Read the model definition and answer for the solid it produces. Units are mm, in the model's axes. A direction names the side the tool comes from. Coordinates: 2 decimals unless noted, no trailing zeros. Write each loop counter-clockwise with the first axis right and the second up, starting at its lowest first coordinate (ties: lowest second). Pieces come first, ordered by that corner, then holes.
Item 1: A tool of negligible diameter and unlimited length cuts with its end or side. For faces 1 (the face through (30, 6, -66.1)), 2 (the face through (73.379, 5.944, -44.985)), 3 (the face through (49, 10, -2)), from which of +Z, -Z, +X, -X, +Y, -Y can it reach the whole face along a straight path? Write none if from no direction.
Item 2: Straight lines are drawn through the part: probe 1 along X at (y, z) = (6.5, -41.3); probe 2 along Z at (x, y) = (88.5, 6.75); probe 3 along Z at (x, y) = (56, 5.5). For each, find the intervals that lie inside material, in ascending order.
Item 3: Section D-D (x = 70) is taken. Give the vertices of the cut face in (y, z).
Item 4: Section C-C (x = 36.5) is taken. Give the vertices of the cut face in (y, z), then the cut area to 3 significant figures.
Item 5: Section A-A (y = 4) is taken. Give the vertices of the cut face in (x, z).
Item 6: Determine the mould class of faces 4 (the face through (69, 10, -44)), 5 (the face through (68.722, 5.36, -42.966)), 6 (the face through (60, 1, -81)) for opening direction X: released by +X, released by -X, zero draft, split by the parting line, or undercut.
Item 7: Section B-B (z = -41.3) is taken. Give the vertices of the cut face in (x, y), then the cut area to 3 significant figures.
Item 8: Each of these flat-tipped pins is pushed along its axis until it touches: P1, Ø1.5, axis at x = 51.5, y = 3.5, coming from the -Z side; P2, Ø2.5, axis at x = 72, z = -86, coming from the +Y side; P3, Ø8, axis at x = 44, z = -55, coming from the +Y side. Where does it stop, or does it pass through?
from build123d import *

# Parameters (mm, degrees)
AUFSATZ_LINEAR_AUSTRAGEN1_DEPTH = 2
SKIZZE2_R                       = 5
SKIZZE2_W                       = 60
SKIZZE2_H                       = 3.5
SKIZZE2_W_2                     = 40
SKIZZE2_W_3                     = 100
AUFSATZ_LINEAR_AUSTRAGEN2_DEPTH = 8
SKIZZE3_R                       = 2.1
SCHNITT_LINEAR_AUSTRAGEN1_DEPTH = 9
FASE1_SIZE                      = 0.4
SKIZZE4_W                       = 58
SKIZZE4_H                       = 1.2
SKIZZE4_W_2                     = 40
SKIZZE4_W_3                     = 100
AUFSATZ_LINEAR_AUSTRAGEN3_DEPTH = 1.6


with BuildPart() as part:
    # Skizze1 → Aufsatz-Linear austragen1 (new body)
    with BuildSketch(Plane(origin=(0, 0, 0), x_dir=(1, 0, 0), z_dir=(0, 1, 0))):
        Polygon((0, 66.1), (0, 0), (100, 0), (100, 88.6), (60, 88.6), (60, 66.1), align=None)
    extrude(amount=AUFSATZ_LINEAR_AUSTRAGEN1_DEPTH)

    # Skizze2 → Aufsatz-Linear austragen2 (add)
    with BuildSketch(Plane(origin=(0, 2, 0), x_dir=(1, 0, 0), z_dir=(0, 1, 0))):
        with Locations(Location((70, 41.3, 0), (0, 0, 270))):
            Circle(SKIZZE2_R)
        with Locations((30, 64.35)):
            Rectangle(SKIZZE2_W, SKIZZE2_H)
        with Locations((80, 86.85)):
            Rectangle(SKIZZE2_W_2, SKIZZE2_H)
        with Locations((50, 1.75)):
            Rectangle(SKIZZE2_W_3, SKIZZE2_H)
    extrude(amount=AUFSATZ_LINEAR_AUSTRAGEN2_DEPTH)

    # Skizze3 → Schnitt-Linear austragen1 (cut)
    with BuildSketch(Plane(origin=(0, 10, 0), x_dir=(1, 0, 0), z_dir=(0, 1, 0))):
        with Locations(Location((70, 41.3, 0), (0, 0, 270))):
            Circle(SKIZZE3_R)
    extrude(amount=-SCHNITT_LINEAR_AUSTRAGEN1_DEPTH, mode=Mode.SUBTRACT)

    # Fase1
    fase1_edges = [part.edges().sort_by_distance(p)[0] for p in [
        (70, 10, -43.4),
    ]]
    chamfer(fase1_edges, length=FASE1_SIZE)

    # Skizze4 → Aufsatz-Linear austragen3 (add)
    with BuildSketch(Plane(origin=(0, 10, 0), x_dir=(1, 0, 0), z_dir=(0, 1, 0))):
        with Locations((29, 65.5)):
            Rectangle(SKIZZE4_W, SKIZZE4_H)
        with Locations((80, 88)):
            Rectangle(SKIZZE4_W_2, SKIZZE4_H)
        with Locations((50, 0.6)):
            Rectangle(SKIZZE4_W_3, SKIZZE4_H)
    extrude(amount=AUFSATZ_LINEAR_AUSTRAGEN3_DEPTH)


solid = part.part
Established:
1. face 1: -Z, -X, +Y, -Y
1. face 2: +Y
1. face 3: +X, -X, +Y
2. probe 1: x = 65 to 67.9, 72.1 to 75
2. probe 2: z = -88.6 to -85.1, -3.5 to 0
2. probe 3: z = -66.1 to -62.6, -3.5 to 0
3. outline: (0, -88.6) - (11.6, -88.6) - (11.6, -87.4) - (10, -87.4) - (10, -85.1) - (2, -85.1) - (2, -46.3) - (10, -46.3) - (10, -43.8) - (9.6, -43.4) - (1, -43.4) - (1, -39.2) - (9.6, -39.2) - (10, -38.8) - (10, -36.3) - (2, -36.3) - (2, -3.5) - (10, -3.5) - (10, -1.2) - (11.6, -1.2) - (11.6, 0) - (0, 0) - close
4. outline: (0, -66.1) - (11.6, -66.1) - (11.6, -64.9) - (10, -64.9) - (10, -62.6) - (2, -62.6) - (2, -3.5) - (10, -3.5) - (10, -1.2) - (11.6, -1.2) - (11.6, 0) - (0, 0) - close
4. area: 192 mm2
5. outline: (0, -66.1) - (60, -66.1) - (60, -62.6) - (0, -62.6) - close; (0, -3.5) - (100, -3.5) - (100, 0) - (0, 0) - close; (60, -88.6) - (100, -88.6) - (100, -85.1) - (60, -85.1) - close; circle Ø10 at (70, -41.3); hole circle Ø4.2 at (70, -41.3)
6. face 4: zero draft
6. face 5: undercut
6. face 6: released by -X
7. outline: (0, 0) - (100, 0) - (100, 2) - (75, 2) - (75, 10) - (72.5, 10) - (72.1, 9.6) - (72.1, 1) - (67.9, 1) - (67.9, 9.6) - (67.5, 10) - (65, 10) - (65, 2) - (0, 2) - close
7. area: 242 mm2
8. P1: stops at z = -66.1
8. P2: stops at y = 10
8. P3: stops at y = 2
